from build123d import *

# Parameters (mm, degrees)
CROQUIS1_R              = 1.7
SALIENTE_EXTRUIR1_DEPTH = 2


with BuildPart() as part:
    # Croquis1 → Saliente-Extruir1 (new body)
    with BuildSketch(Plane(origin=(0, 0, 0), x_dir=(1, 0, 0), z_dir=(0, 1, 0))):
        Polygon((-8.046684223, -2.46171515), (-8.046684223, 2.46171515), (-8.046684223, 6), (8.046684223, 6), (8.046684223, 2.46171515), (8.046684223, -2.46171515), (8.046684223, -6), (-8.046684223, -6), align=None)
        with BuildLine():
            Line((8.046684223, -2.46171515), (8.046684223, 2.46171515))
            ThreePointArc((8.046684223, 2.46171515), (8.827888747, 2.181898598), (9.657649034, 2.173199442))
            ThreePointArc((9.657649034, 2.173199442), (12.2, 0), (9.657649034, -2.173199442))
            ThreePointArc((9.657649034, -2.173199442), (8.827888747, -2.181898598), (8.046684223, -2.46171515))
        make_face()
        with Locations((10, 0)):
            Circle(CROQUIS1_R, mode=Mode.SUBTRACT)
        with BuildLine():
            ThreePointArc((-9.657649034, -2.173199442), (-12.2, 0), (-9.657649034, 2.173199442))
            ThreePointArc((-9.657649034, 2.173199442), (-8.827888747, 2.181898598), (-8.046684223, 2.46171515))
            Line((-8.046684223, 2.46171515), (-8.046684223, -2.46171515))
            ThreePointArc((-8.046684223, -2.46171515), (-8.827888747, -2.181898598), (-9.657649034, -2.173199442))
        make_face()
        with Locations((-10, 0)):
            Circle(CROQUIS1_R, mode=Mode.SUBTRACT)
        with BuildLine():
            Line((-8.046684223, -6), (-8.046684223, -2.46171515))
            ThreePointArc((-8.046684223, -2.46171515), (-8.827888747, -2.181898598), (-9.657649034, -2.173199442))
            ThreePointArc((-9.657649034, -2.173199442), (-11.429480303, -1.672299633), (-12.2, 0))
            Line((-12.2, 0), (-12.2, -6))
            Line((-12.2, -6), (-8.046684223, -6))
        make_face()
        with BuildLine():
            Line((-8.046684223, 2.46171515), (-8.046684223, 6))
            Line((-8.046684223, 6), (-12.2, 6))
            Line((-12.2, 6), (-12.2, 0))
            ThreePointArc((-12.2, 0), (-11.429480303, 1.672299633), (-9.657649034, 2.173199442))
            ThreePointArc((-9.657649034, 2.173199442), (-8.827888747, 2.181898598), (-8.046684223, 2.46171515))
        make_face()
        with BuildLine():
            Line((12.2, 6), (8.046684223, 6))
            Line((8.046684223, 6), (8.046684223, 2.46171515))
            ThreePointArc((8.046684223, 2.46171515), (8.827888747, 2.181898598), (9.657649034, 2.173199442))
            ThreePointArc((9.657649034, 2.173199442), (11.429480303, 1.672299633), (12.2, 0))
            Line((12.2, 0), (12.2, 6))
        make_face()
        with BuildLine():
            ThreePointArc((9.657649034, -2.173199442), (8.827888747, -2.181898598), (8.046684223, -2.46171515))
            Line((8.046684223, -2.46171515), (8.046684223, -6))
            Line((8.046684223, -6), (12.2, -6))
            Line((12.2, -6), (12.2, 0))
            ThreePointArc((12.2, 0), (11.429480303, -1.672299633), (9.657649034, -2.173199442))
        make_face()
    extrude(amount=SALIENTE_EXTRUIR1_DEPTH)


solid = part.part
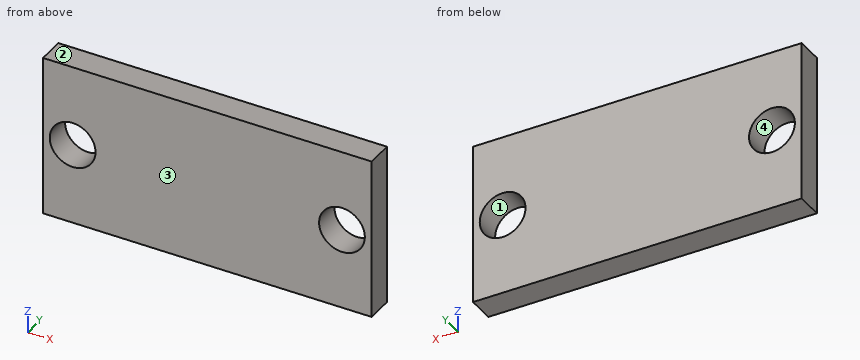
CAD build for the part. Positions are in the model's coordinates, mm. Face numbers are marked on the shaded views. Coordinates: 2 decimals unless noted, no trailing zeros. Write each loop counter-clockwise with the first axis right and the second up, starting at its lowest first coordinate (ties: lowest second). Pieces come first, ordered by that corner, then holes. Notation, with made-up numbers: (9.25, 82) - (34.25, 82) arc R25 ccw to (34.25, 102) - close; hole circle Ø5 at (31, 9). An arc over 180 degrees is marked (long way). Use a Markdown table: item, result. Add a question column.
Item 1: Band-saw the part on A-A, the plane z = 0. Give the cut face in (x, y).
Item 2: Band-saw the part on D-D, the plane x = 9.5. Give the cut face in (y, z).
Item 3: Band-saw the part on C-C, the plane y = 1.6. Give the cut face in (x, z), and give its area (3 significant figures).
Item 4: Mould opens along Z. For the marked faces 1, 2, 3 and 4 say: pulls with the +Z half, pulls with the -Z half, needs draft (parallel to the pull), parting line crosses it, or undercut.
Item 5: Band-saw the part on B-B, the plane x = -10. Give the cut face in (y, z).
Item 6: Drill centre lines: L1, parallel to X at y = 1.25, z = 0; L2, parallel to Z at x = -10, y = 0.4; L3, parallel to X at y = 0.6, z = -0.75. Where is each one in solid material? Low to high. Write a range as from..to.
Numbers:
| question | item | result |
|---|---|---|
| 1 | outline | (-12.2, 0) - (-11.7, 0) - (-11.7, 2) - (-12.2, 2) - close; (-8.3, 0) - (8.3, 0) - (8.3, 2) - (-8.3, 2) - close; (11.7, 0) - (12.2, 0) - (12.2, 2) - (11.7, 2) - close |
| 2 | outline | (0, -6) - (2, -6) - (2, -1.62) - (0, -1.62) - close; (0, 1.62) - (2, 1.62) - (2, 6) - (0, 6) - close |
| 3 | outline | (-12.2, -6) - (12.2, -6) - (12.2, 6) - (-12.2, 6) - close; hole circle Ø3.4 at (-10, 0); hole circle Ø3.4 at (10, 0) |
| 3 | area | 275 mm2 |
| 4 | face 1 | undercut |
| 4 | face 2 | pulls with the +Z half |
| 4 | face 3 | needs draft |
| 4 | face 4 | undercut |
| 5 | outline | (0, -6) - (2, -6) - (2, -1.7) - (0, -1.7) - close; (0, 1.7) - (2, 1.7) - (2, 6) - (0, 6) - close |
| 6 | L1 | -12.2..-11.7, -8.3..8.3, 11.7..12.2 |
| 6 | L2 | -6..-1.7, 1.7..6 |
| 6 | L3 | -12.2..-11.53, -8.47..8.47, 11.53..12.2 |
